from build123d import *

# Parameters (mm, degrees)
SKETCH2_W           = 50
SKETCH2_H           = 50
BOSS_EXTRUDE4_DEPTH = 10
SKETCH5_W           = 50
SKETCH5_H           = 50
BOSS_EXTRUDE5_DEPTH = 50
SKETCH6_W           = 50
SKETCH6_H           = 50
BOSS_EXTRUDE6_DEPTH = 100
SKETCH7_W           = 50
SKETCH7_H           = 50
BOSS_EXTRUDE7_DEPTH = 100
SKETCH8_W           = 50
SKETCH8_H           = 50
BOSS_EXTRUDE8_DEPTH = 50


with BuildPart() as part:
    # Sketch2 → Boss-Extrude4 (new body)
    with BuildSketch(Plane(origin=(0, 0, 0), x_dir=(1, 0, 0), z_dir=(0, 1, 0))):
        Polygon((-125, 75), (-175, 75), (-175, 25), (-225, 25), (-225, -25), (-175, -25), (-175, -75), (-125, -75), (-125, -25), (-75, -25), (-75, -75), (-25.420673077, -75), (-25.420673077, -25), (24.579326923, -25), (24.579326923, -75), (75, -75), (75, -25), (125, -25), (125, -75), (175, -75), (175, -25), (225, -25), (225, 25), (175, 25), (175, 75), (125, 75), (125, 25), (75, 25), (75, 75), (24.579326923, 75), (24.579326923, 25), (-25.420673077, 25), (-25.420673077, 75), (-75, 75), (-75, 25), (-125, 25), align=None)
        with Locations((-200, -50)):
            Rectangle(SKETCH2_W, SKETCH2_H)
        with Locations((-100, -50)):
            Rectangle(SKETCH2_W, SKETCH2_H)
        with Locations((-200, 50)):
            Rectangle(SKETCH2_W, SKETCH2_H)
        with Locations((-100, 50)):
            Rectangle(SKETCH2_W, SKETCH2_H)
        with Locations((-0.420673077, -50)):
            Rectangle(SKETCH2_W, SKETCH2_H)
        with Locations((-0.420673077, 50)):
            Rectangle(SKETCH2_W, SKETCH2_H)
        with Locations((100, 50)):
            Rectangle(SKETCH2_W, SKETCH2_H)
        with Locations((100, -50)):
            Rectangle(SKETCH2_W, SKETCH2_H)
        with Locations((200, -50)):
            Rectangle(SKETCH2_W, SKETCH2_H)
        with Locations((200, 50)):
            Rectangle(SKETCH2_W, SKETCH2_H)
    extrude(amount=BOSS_EXTRUDE4_DEPTH)

    # Sketch5 → Boss-Extrude5 (add)
    with BuildSketch(Plane(origin=(0, 10, 0), x_dir=(1, 0, 0), z_dir=(0, 1, 0))):
        with Locations((-200, 50)):
            Rectangle(SKETCH5_W, SKETCH5_H)
        with Locations((200, 50)):
            Rectangle(SKETCH5_W, SKETCH5_H)
    extrude(amount=BOSS_EXTRUDE5_DEPTH)

    # Sketch6 → Boss-Extrude6 (add)
    with BuildSketch(Plane(origin=(0, 10, 0), x_dir=(1, 0, 0), z_dir=(0, 1, 0))):
        with Locations((-200, -50)):
            Rectangle(SKETCH6_W, SKETCH6_H)
        with Locations((200, -50)):
            Rectangle(SKETCH6_W, SKETCH6_H)
    extrude(amount=BOSS_EXTRUDE6_DEPTH)

    # Sketch7 → Boss-Extrude7 (add)
    with BuildSketch(Plane(origin=(0, 10, 0), x_dir=(1, 0, 0), z_dir=(0, 1, 0))):
        with Locations((-100, 50)):
            Rectangle(SKETCH7_W, SKETCH7_H)
        with Locations((0, 50)):
            Rectangle(SKETCH7_W, SKETCH7_H)
        with Locations((100, 50)):
            Rectangle(SKETCH7_W, SKETCH7_H)
    extrude(amount=BOSS_EXTRUDE7_DEPTH)

    # Sketch8 → Boss-Extrude8 (add)
    with BuildSketch(Plane(origin=(0, 10, 0), x_dir=(1, 0, 0), z_dir=(0, 1, 0))):
        with Locations((-100, -50)):
            Rectangle(SKETCH8_W, SKETCH8_H)
        with Locations((0, -50)):
            Rectangle(SKETCH8_W, SKETCH8_H)
        with Locations((100, -50)):
            Rectangle(SKETCH8_W, SKETCH8_H)
    extrude(amount=BOSS_EXTRUDE8_DEPTH)


solid = part.part
Read the model definition and answer for the solid it produces. Units are mm, in the model's axes. A direction names the side the tool comes from. Coordinates: 2 decimals unless noted, no trailing zeros. Loops run counter-clockwise (first coordinate to the right, second up) from the corner with the lowest first, then second, coordinate; pieces in that order, holes last.
Q1. Consider probe 1 along X at (y, z) = (64.5, -26); probe 2 along X at (y, z) = (26.5, 29); probe 3 along Z at (x, y) = (-108, 18). Determine where each line is inside the solid, lowest interval first.
Q2. The part is cut by section A-A on y = 84. Write down the section's boundary in (x, z), and give its area (3 significant figures).
Q3. Each of these flat-tipped pins is pushed along its axis until it touches: pin 1 Ø15 at (x, z) = (-101.5, 44) entering from +Y; pin 2 Ø2 at (x, z) = (-38, -36) entering from +Y. Where does it stop, or does it pass through?
Q4. The part is cut by section C-C on y = 42. Give the number of separate pieces and of enclosed holes in the cut face, and give its area (3 significant figures).
Q5. The part is cut by section B-B on z = -47. Write down the section's boundary in (x, y).
Q6. The part is cut by section D-D on x = -145. Write down the section's boundary in (y, z).
Q7. The mould has two halves that part along X. Classify faces 1 (the face through (0, 59, -25)), 2 (the face through (-175, 35, -50)): +X half, -X half, draft (parallel to the pull), parting line (faces both ways), or undercut.
Q8. Which of the six approach directions +Z, -Z, +X, -X, +Y, -Y give full straight-line access (tool end or side, diameter ignored) to faces 3 (the face through (-100, 35, 25)), 4 (the face through (-100, 60, 50)), 5 (the face through (-200, 60, -50)), 6 (the face through (-3, 0, -1)), 7 (the face through (-75, 59, -50))?
Results below:
1. probe 1: x = -125 to -75, -25 to 25, 75 to 125
1. probe 2: x = -225 to -175, -125 to -75, -25 to 25, 75 to 125, 175 to 225
1. probe 3: z = -75 to -25, 25 to 75
2. outline: (-225, 25) - (-175, 25) - (-175, 75) - (-225, 75) - close; (-125, -75) - (-75, -75) - (-75, -25) - (-125, -25) - close; (-25, -75) - (25, -75) - (25, -25) - (-25, -25) - close; (75, -75) - (125, -75) - (125, -25) - (75, -25) - close; (175, 25) - (225, 25) - (225, 75) - (175, 75) - close
2. area: 12,500 mm2
3. pin 1: stops at y = 60
3. pin 2: stops at y = 10
4. separate pieces: 10
4. enclosed holes: 0
4. area: 25,000 mm2
5. outline: (-225, 0) - (225, 0) - (225, 60) - (175, 60) - (175, 10) - (125, 10) - (125, 110) - (75, 110) - (75, 10) - (25, 10) - (25, 110) - (-25, 110) - (-25, 10) - (-75, 10) - (-75, 110) - (-125, 110) - (-125, 10) - (-175, 10) - (-175, 60) - (-225, 60) - close
6. outline: (0, -75) - (10, -75) - (10, 75) - (0, 75) - close
7. face 1: draft
7. face 2: undercut
8. face 3: +X, -X, +Y
8. face 4: +Z, +Y
8. face 5: -Z, -X, +Y
8. face 6: +Z, -Z, +X, -X, -Y
8. face 7: +Z, -Z, +Y
